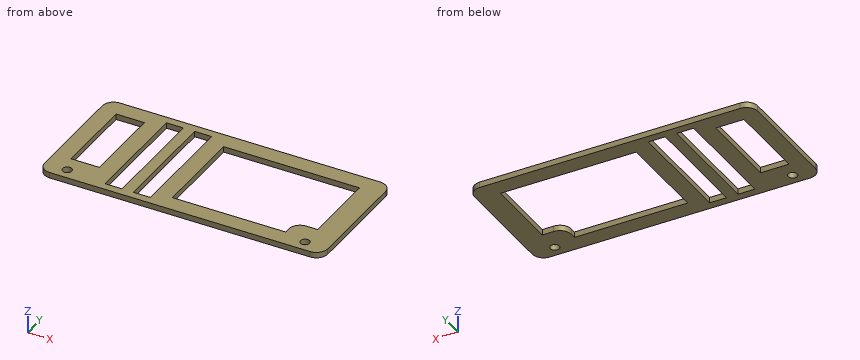
```python
from build123d import *

# Parameters (mm, degrees)
SKETCH1_W           = 250
SKETCH1_H           = 112
BOSS_EXTRUDE1_DEPTH = 5
SKETCH2_R           = 4
CUT_EXTRUDE1_DEPTH  = 11
SKETCH3_R           = 4
CUT_EXTRUDE2_DEPTH  = 15
SKETCH4_W           = 15
SKETCH4_H           = 98
CUT_EXTRUDE4_DEPTH  = 15
CUT_EXTRUDE5_DEPTH  = 15
FILLET1_R           = 10
SKETCH6_W           = 25
SKETCH6_H           = 72
CUT_EXTRUDE6_DEPTH  = 5


with BuildPart() as part:
    # Sketch1 → Boss-Extrude1 (new body)
    with BuildSketch(Plane.XY):
        with Locations((-57.664233577, 31.912408759)):
            Rectangle(SKETCH1_W, SKETCH1_H)
    extrude(amount=BOSS_EXTRUDE1_DEPTH)

    # Sketch2 → Cut-Extrude1 (cut)
    with BuildSketch(Plane.XY.offset(5)):
        with Locations((-162.664233577, -14.087591241)):
            Circle(SKETCH2_R)
    extrude(amount=-CUT_EXTRUDE1_DEPTH, mode=Mode.SUBTRACT)

    # Sketch3 → Cut-Extrude2 (cut)
    with BuildSketch(Plane.XY.offset(5)):
        with Locations((47.335766423, -14.087591241)):
            Circle(SKETCH3_R)
    extrude(amount=-CUT_EXTRUDE2_DEPTH, mode=Mode.SUBTRACT)

    # Sketch4 → Cut-Extrude4 (cut)
    with BuildSketch(Plane.XY.offset(5)):
        with Locations((-120.164233577, 31.912408759)):
            Rectangle(SKETCH4_W, SKETCH4_H)
        with Locations((-95.164233577, 31.912408759)):
            Rectangle(SKETCH4_W, SKETCH4_H)
    extrude(amount=-CUT_EXTRUDE4_DEPTH, mode=Mode.SUBTRACT)

    # Sketch5 → Cut-Extrude5 (cut)
    with BuildSketch(Plane.XY.offset(5)):
        Polygon((17.397729683, 72.912408759), (-72.664233577, 72.912408759), (-72.664233577, -9.087591241), (27.335766423, -9.087591241), (27.335766423, 5.912408759), (47.335766423, 5.912408759), (47.335766423, 72.912408759), align=None)
    extrude(amount=-CUT_EXTRUDE5_DEPTH, mode=Mode.SUBTRACT)

    # Fillet1
    fillet1_edges = [part.edges().sort_by_distance(p)[0] for p in [
        (27.335766423, 5.912408759, 2.5),
        (-182.664233577, 87.912408759, 2.5),
        (67.335766423, 87.912408759, 2.5),
        (67.335766423, -24.087591241, 2.5),
        (-182.664233577, -24.087591241, 2.5),
    ]]
    fillet(fillet1_edges, radius=FILLET1_R)

    # Sketch6 → Cut-Extrude6 (cut)
    with BuildSketch(Plane.XY.offset(5)):
        with Locations((-155.164233577, 36.912408759)):
            Rectangle(SKETCH6_W, SKETCH6_H)
    extrude(amount=-CUT_EXTRUDE6_DEPTH, mode=Mode.SUBTRACT)


solid = part.part
```
The listing builds one solid part. Answer for the finished solid, in the listing's coordinates (mm). Coordinates: 2 decimals unless noted, no trailing zeros. Write each loop counter-clockwise with the first axis right and the second up, starting at its lowest first coordinate (ties: lowest second). Pieces come first, ordered by that corner, then holes. Notation, with made-up numbers: (60.25, 40) - (82.25, 40) arc R27 ccw to (82.25, 71) - close; hole circle Ø11 at (10.25, 23). An arc over 180 degrees is marked (long way). Return JSON: item names as keys, results as strings. Group by question number.
Q1. The part is cut by section C-C on y = 64. Write down the section's boundary in (x, z).
Q2. A flat-ended cylindrical pin translates along its axis: pin 1 Ø1.5 at (x, y) = (-11, -10) entering from -Z. Find the tip coordinate at first contact, or state that the pin passes through.
Q3. Find the intervals of material crossed by line 1 along X through (y, z) = (53, 3.1); line 2 along X through (y, z) = (-13.5, 0.3); line 3 along Y through (x, z) = (21, 0.85), in increasing order. Write a range as [from, to].
Q4. The part is cut by section B-B on z = 3.05. State how many separate pieces and enclosed holes the cut face has, and give its area (3 significant figures).
Q5. The part is cut by section A-A on x = 11. Write down the section's boundary in (y, z), and give its area (3 significant figures).
Evaluation:
{
 "1": {"outline": "(-182.66, 0) - (-167.66, 0) - (-167.66, 5) - (-182.66, 5) - close; (-142.66, 0) - (-127.66, 0) - (-127.66, 5) - (-142.66, 5) - close; (-112.66, 0) - (-102.66, 0) - (-102.66, 5) - (-112.66, 5) - close; (-87.66, 0) - (-72.66, 0) - (-72.66, 5) - (-87.66, 5) - close; (47.34, 0) - (67.34, 0) - (67.34, 5) - (47.34, 5) - close"},
 "2": {"pin 1": "stops at z = 0"},
 "3": {"line 1": "x = [-182.66, -167.66], [-142.66, -127.66], [-112.66, -102.66], [-87.66, -72.66], [47.34, 67.34]", "line 2": "x = [-182.66, -166.62], [-158.71, -127.66], [-112.66, -102.66], [-87.66, 43.38], [51.29, 67.34]", "line 3": "y = [-24.09, -9.09], [72.91, 87.91]"},
 "4": {"separate pieces": "1", "enclosed holes": "6", "area": "13,500 mm2"},
 "5": {"outline": "(-24.09, 0) - (-9.09, 0) - (-9.09, 5) - (-24.09, 5) - close; (72.91, 0) - (87.91, 0) - (87.91, 5) - (72.91, 5) - close", "area": "150 mm2"}
}
